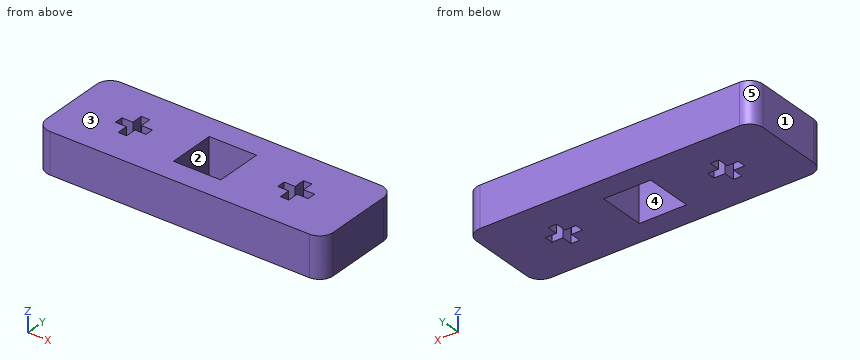
from build123d import *

# Parameters (mm, degrees)
SKETCH_W   = 42.2
SKETCH_H   = 13.8
SKETCH_W_2 = 6.95
SKETCH_H_2 = 6.95
PAD_DEPTH  = 6
FILLET_R   = 2


with BuildPart() as part:
    # Sketch → Pad (new body)
    with BuildSketch(Plane.XY):
        Rectangle(SKETCH_W, SKETCH_H)
        Rectangle(SKETCH_W_2, SKETCH_H_2, mode=Mode.SUBTRACT)
        Polygon((9.687999, 0.625), (9.687999, -0.625), (11.312999, -0.625), (11.312999, -2.25), (12.562999, -2.25), (12.562999, -0.625), (14.187999, -0.625), (14.187999, 0.625), (12.562999, 0.625), (12.562999, 2.25), (11.312999, 2.25), (11.312999, 0.625), align=None, mode=Mode.SUBTRACT)
        Polygon((-14.187999, 0.625), (-14.188001, -0.625), (-12.563001, -0.625), (-12.563001, -2.25), (-11.313001, -2.25), (-11.313001, -0.625), (-9.687999, -0.625), (-9.687999, 0.625), (-11.312999, 0.625), (-11.312999, 2.25), (-12.562999, 2.25), (-12.562999, 0.625), align=None, mode=Mode.SUBTRACT)
    extrude(amount=PAD_DEPTH)

    # Fillet
    fillet_edges = [part.edges().sort_by_distance(p)[0] for p in [
        (21.1, -6.9, 3),
        (21.1, 6.9, 3),
        (-21.1, -6.9, 3),
        (-21.1, 6.9, 3),
    ]]
    fillet(fillet_edges, radius=FILLET_R)


solid = part.part
Read the model definition and answer for the solid it produces. Units are mm, in the model's axes. Face numbers are marked on the shaded views. A direction names the side the tool comes from. Round coordinates to 2 decimals unless told otherwise and drop trailing zeros. Write each loop counter-clockwise with the first axis right and the second up, starting at its lowest first coordinate (ties: lowest second). Pieces come first, ordered by that corner, then holes. Notation, with made-up numbers: (-13.75, 33) - (28.25, 33) arc R17 cw to (28.25, 50) - close; hole circle Ø2 at (10, 44.5). An arc over 180 degrees is marked (long way). Use a Markdown table: item, result.
(1) The part is cut by section D-D (z = 5.4). State how many separate pieces and enclosed holes the cut face has, then the cut area to 3 significant figures.
Reported:
| item | result |
|---|---|
| separate pieces | 1 |
| enclosed holes | 3 |
| area | 511 mm2 |
(2) The part is cut by section A-A (y = -3). Write down the section's boundary in (x, z) (3 decimals), then the cut area to 4 significant figures.
Reported:
| item | result |
|---|---|
| outline | (-21.1, 0) - (-3.475, 0) - (-3.475, 6) - (-21.1, 6) - close; (3.475, 0) - (21.1, 0) - (21.1, 6) - (3.475, 6) - close |
| area | 211.5 mm2 |
(3) The mould has two halves that part along Y. Classify the marked faces 3, 4 and 5: released by +Y, released by -Y, zero draft, split by the parting line, or undercut.
Reported:
| item | result |
|---|---|
| face 3 | zero draft |
| face 4 | undercut |
| face 5 | released by +Y |
(4) Straight lines are drawn through the part: line 1 along X through (y, z) = (1.5, 1.5) (3 decimals); line 2 along Y through (x, z) = (-2.5, 5.45) (3 decimals); line 3 along X through (y, z) = (3.25, 4.3) (3 decimals). For each, find the intervals that lie inside material, in ascending order. Write a range as [from, to].
Reported:
| item | result |
|---|---|
| line 1 | [-21.1, -12.563], [-11.313, -3.475], [3.475, 11.313], [12.563, 21.1] |
| line 2 | [-6.9, -3.475], [3.475, 6.9] |
| line 3 | [-21.1, -3.475], [3.475, 21.1] |
(5) The part is cut by section B-B (x = 2.5). Write down the section's boundary in (y, z) (3 decimals), then the cut area to 3 significant figures.
Reported:
| item | result |
|---|---|
| outline | (-6.9, 0) - (-3.475, 0) - (-3.475, 6) - (-6.9, 6) - close; (3.475, 0) - (6.9, 0) - (6.9, 6) - (3.475, 6) - close |
| area | 41.1 mm2 |
(6) Which of the six approach directions +Z, -Z, +X, -X, +Y, -Y give full straight-line access (tool end or side, diameter ignored) to the marked faces 1 and 2?
Reported:
| item | result |
|---|---|
| face 1 | +Z, -Z, -X, +Y, -Y |
| face 2 | +Z, -Z |
(7) The part is cut by section C-C (y = 1). Write down the section's boundary in (x, z) (3 decimals).
Reported:
| item | result |
|---|---|
| outline | (-21.1, 0) - (-12.563, 0) - (-12.563, 6) - (-21.1, 6) - close; (-11.313, 0) - (-3.475, 0) - (-3.475, 6) - (-11.313, 6) - close; (3.475, 0) - (11.313, 0) - (11.313, 6) - (3.475, 6) - close; (12.563, 0) - (21.1, 0) - (21.1, 6) - (12.563, 6) - close |
